Read the model definition and answer for the solid it produces. Units are mm, in the model's axes. Face numbers are marked on the shaded views. A direction names the side the tool comes from. Coordinates: 2 decimals unless noted, no trailing zeros. Order: outer loops, then holes, each group sorted by start corner. A loop starts at its lowest first (then second) coordinate and runs counter-clockwise, first axis right, second up.
Autodesk Inventor part; units mm, degrees
ref_plane "YZ Plane" through (0, 0, 0) normal (1, 0, 0) x (0, 1, 0)
ref_plane "XZ Plane" through (0, 0, 0) normal (0, 1, 0) x (-1, 0, 0)
ref_plane "XY Plane" through (0, 0, 0) normal (0, 0, 1) x (1, 0, 0)
sketch "Sketch1" plane through (0, 0, 0) normal (0, 0, 1) x (1, 0, 0)
  line L0 (-21.15, -21.15) -> (21.15, -21.15) construction
  line L1 (21.15, -21.15) -> (21.15, 21.15)
  line L2 (21.15, 21.15) -> (-21.15, 21.15)
  line L3 (-21.15, 21.15) -> (-21.15, -21.15)
  line L4 (-21.15, -21.15) -> (21.15, 21.15) construction
  line L5 (21.15, -21.15) -> (-21.15, 21.15) construction
  line L6 (15.5, 15.5) -> (-15.5, 15.5) construction
  line L7 (-15.5, 15.5) -> (-15.5, -15.5) construction
  line L8 (-15.5, -15.5) -> (15.5, -15.5) construction
  line L9 (15.5, -15.5) -> (15.5, 15.5) construction
  line L10 (15.5, 15.5) -> (-15.5, -15.5) construction
  line L11 (-15.5, 15.5) -> (15.5, -15.5) construction
  line L12 (-21.15, -21.15) -> (-21.15, -44.15)
  line L13 (-21.15, -44.15) -> (21.15, -44.15)
  line L14 (21.15, -44.15) -> (21.15, -21.15)
  line L15 (21.15, -34.15) -> (-21.15, -34.15) construction
  circle A0 centre (-13.15, -34.15) radius 2.75
  circle A1 centre (13.15, -34.15) radius 2.75
  circle A2 centre (0, 0) radius 11.5
  circle A3 centre (-15.5, -15.5) radius 1.75
  circle A4 centre (15.5, -15.5) radius 1.75
  circle A5 centre (-15.5, 15.5) radius 1.75
  circle A6 centre (15.5, 15.5) radius 1.75
  dimension "d0" = 42.3
  dimension "d1" = 42.3
  dimension "d2" = 10
  dimension "d3" = 23
  dimension "d4" = 8
  dimension "d5" = 8
  dimension "d6" = 5.5
  dimension "d7" = 31
  dimension "d8" = 3.5
  dimension "d9" = 23
extrude "Extrusion1" add sketch "Sketch1" along normal blind 2.5
sketch "Sketch2" plane through (21.15, -44.15, 0) normal (1, 0, 0) x (0, 0, -1)
  line L0 (0, 0) -> (-2.5, 0) construction
  line L1 (0, 65.3) -> (-2.5, 65.3) construction
  line L2 (-2.5, 0) -> (-2.5, 65.3) construction
  line L3 (-2.5, 65.3) -> (0, 65.3) construction
  line L4 (0, 65.3) -> (20.3, 22) construction
  line L5 (20.3, 22) -> (20.3, 0)
  line L6 (20.3, 0) -> (-2.5, 0) construction
  line L7 (20.3, 22) -> (0, 22)
  line L8 (0, 22) -> (0, 65.3)
  line L9 (20.3, 0) -> (22.8, 0)
  line L10 (22.8, 0) -> (22.8, 22)
  line L11 (0, 0) -> (0, 65.3)
  line L12 (22.8, 22) -> (0, 65.3)
  line L13 (20.3, 22) -> (22.8, 22) construction
  line L14 (0, 0) -> (0, 65.3)
  line L15 (0, 65.3) -> (-2.5, 65.3)
  line L16 (-2.5, 0) -> (-2.5, 65.3)
  line L17 (0, 0) -> (-2.5, 0)
  point P0 (0, 44.15)
  point P1 (0, 65.3)
  dimension "d12" = 22
  dimension "d14" = 2.5
  dimension "d28" = 20.3
extrude "Extrusion2" add sketch "Sketch2" along normal blind 3
mirror "Mirror1" about plane through (0, 0, 0) normal (1, 0, 0) of "Extrusion2"
sketch "Sketch3" plane through (-21.15, -44.15, -20.3) normal (1, 0, 0) x (0, 0, -1)
  line L0 (0, 22) -> (0, 0)
  line L1 (0, 22) -> (2.5, 22)
  line L2 (2.5, 22) -> (2.5, 0)
  line L3 (2.5, 0) -> (0, 0)
  line L4 (0, 0) -> (0, 22)
  point P0 (-20.3, 44.15)
extrude "Extrusion3" add sketch "Sketch3" along normal up to surface (42.3 mm away)
sketch "Sketch4" plane through (24.15, -44.15, -20.3) normal (0, 0, 1) x (1, 0, 0)
  line L0 (-45.3, 22) -> (-48.3, 22)
  line L1 (0, 22) -> (0, 0)
  line L2 (-48.3, 22) -> (0, 22)
  line L3 (0, 22) -> (0, 20)
  line L4 (0, 20) -> (-48.3, 20)
  line L5 (-48.3, 20) -> (-48.3, 22)
  point P0 (-24.15, 44.15)
  point P1 (0, 22)
  dimension "d19" = 2
extrude "Extrusion4" add sketch "Sketch4" along normal up to surface (20.3 mm away)
sketch "Sketch5" plane through (24.15, -44.15, -22.8) normal (0, 0, -1) x (-1, 0, 0)
  line L0 (48.3, 0) -> (0, 0)
  line L1 (24.15, 0) -> (24.15, 10) construction
  circle A0 centre (24.15, 10) radius 2.75
  point P0 (24.15, 44.15)
  dimension "d22" = 5.5
  dimension "d23" = 10
extrude "Extrusion5" cut sketch "Sketch5" against normal up to surface (2.5 mm away)
fillet "Fillet1" radius 10 2 edges at (24.15, -44.15, -21.55) (-24.15, -44.15, -21.55)
fillet "Fillet1" radius 4 4 edges at (-24.15, -44.15, 1.25) (24.15, -44.15, 1.25) (24.15, 21.15, 1.25) (-24.15, 21.15, 1.25)
properties part number "MotorBracket1"
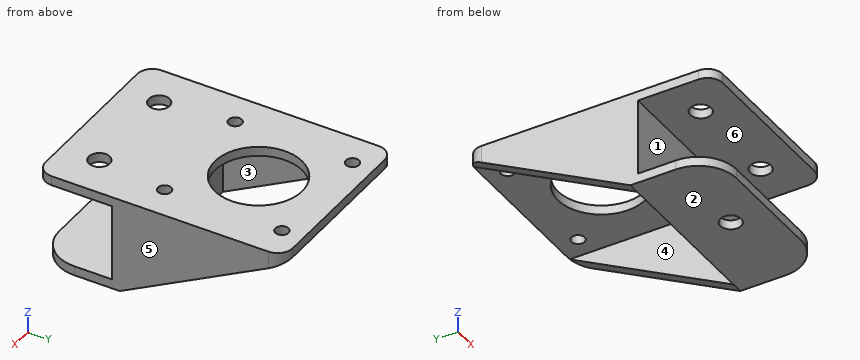
1) A cutting plane is placed at A-A, the plane x = 0. Determine the outline of the cut face in (y, z).
A:
outline: (-44.15, -22.8) - (-36.9, -22.8) - (-36.9, -20.3) - (-44.15, -20.3) - close; (-44.15, 0) - (-24.15, 0) - (-24.15, -20.3) - (-31.4, -20.3) - (-31.4, -22.8) - (-22.15, -22.8) - (-22.15, 0) - (-11.5, 0) - (-11.5, 2.5) - (-44.15, 2.5) - close; (11.5, 0) - (21.15, 0) - (21.15, 2.5) - (11.5, 2.5) - close
2) Determine the mould class of the marked faces 4, 5 and 6 for opening direction X: pulls with the +X half, pulls with the -X half, needs draft (parallel to the pull), parting line crosses it, or undercut.
A:
face 4: undercut
face 5: pulls with the +X half
face 6: needs draft
3) A cutting plane is placed at D-D, the plane x = 7.5. Determine the outline of the cut face in (y, z), and give its area (3 significant figures).
A:
outline: (-44.15, -22.8) - (-22.15, -22.8) - (-22.15, 0) - (-8.72, 0) - (-8.72, 2.5) - (-44.15, 2.5) - (-44.15, 0) - (-24.15, 0) - (-24.15, -20.3) - (-44.15, -20.3) - close; (8.72, 0) - (21.15, 0) - (21.15, 2.5) - (8.72, 2.5) - close
area: 215 mm2
4) A cutting plane is placed at B-B, the plane y = -4. Determine the outline of the cut face in (x, z), and give its area (3 significant figures).
A:
outline: (-24.15, -13.24) - (-21.15, -13.24) - (-21.15, 0) - (-10.78, 0) - (-10.78, 2.5) - (-24.15, 2.5) - close; (10.78, 0) - (21.15, 0) - (21.15, -13.24) - (24.15, -13.24) - (24.15, 2.5) - (10.78, 2.5) - close
area: 146 mm2
5) A cutting plane is placed at C-C, the plane z = -6.5. Determine the outline of the cut face in (x, y).
A:
outline: (-24.15, -24.15) - (24.15, -24.15) - (24.15, 8.81) - (21.15, 8.81) - (21.15, -22.15) - (-21.15, -22.15) - (-21.15, 8.81) - (-24.15, 8.81) - close
6) Which of the six approach directions +Z, -Z, +X, -X, +Y, -Y give full straight-line access (tool end or side, diameter ignored) to the marked faces 1, 2 and 3?
A:
face 1: +X, -X, -Y
face 2: -Z, +X, -X, +Y, -Y
face 3: -Z, +Y
7) Straight lines are drawn through the part: line 1 (Y direction, x = -13.15, z = 1.45); line 2 (X direction, y = -20, z = -16); line 3 (Y direction, x = -15.5, z = 0.8). For each, find the intervals that lie inside material, in ascending order.
A:
line 1: y = -44.15 to -36.9, -31.4 to 21.15
line 2: x = -24.15 to -21.15, 21.15 to 24.15
line 3: y = -44.15 to -35.58, -32.72 to -17.25, -13.75 to 13.75, 17.25 to 21.15
8) Flat-ended cylindrical pins translate along their axes: pin 1 Ø11.5 at (x, z) = (-2.5, -13) entering from +Y; pin 2 Ø3 at (x, y) = (-15.5, -15.5) entering from +Z; pin 3 Ø4 at (x, y) = (15.5, 15.5) entering from -Z; pin 4 Ø6 at (x, z) = (-2, -15) entering from -Y. Find the tip coordinate at first contact, or state that the pin passes through.
A:
pin 1: stops at y = -22.15
pin 2: passes through
pin 3: stops at z = 0
pin 4: stops at y = -24.15
